```python
from build123d import *

# Parameters (mm, degrees)
F0_R      = 3.175
F1_DEPTH  = 38.1
F3_R      = 9.525
F4_DEPTH  = 3.175
F5_R      = 3.048
F6_DEPTH  = 92.0760001
F8_DEPTH  = 6.3510001273
F12_R     = 0.79375
F15_ANGLE = 180


with BuildPart() as f1:
    # F0 (on Top) → F1 (new body, symmetric)
    with BuildSketch(Plane.XY):
        Circle(F0_R)
    extrude(amount=F1_DEPTH, both=True)

    # F3 (on Right) → F4 (join, symmetric)
    with BuildSketch(Plane.YZ):
        with Locations((0, -44.45)):
            Circle(F3_R)
    extrude(amount=F4_DEPTH, both=True)

    # F5 (on face) → F6 (cut, through all)
    with BuildSketch(Plane.XY.offset(38.1)):
        Circle(F5_R)
    extrude(amount=-F6_DEPTH, mode=Mode.SUBTRACT)

    # F7 (on face) → F8 (cut, through all)
    with BuildSketch(Plane.YZ.offset(3.175)):
        with BuildLine():
            ThreePointArc((0, -35.56), (-6.2861792847, -50.7361792847), (8.89, -44.45))
            ThreePointArc((8.89, -44.45), (6.2861792847, -38.1638207153), (0, -35.56))
        make_face()
    extrude(amount=-F8_DEPTH, mode=Mode.SUBTRACT)

    # F12 (on offset) → F13 (join, up to the next surface of F1)
    with BuildSketch(Plane.XZ.offset(9.525)):
        with Locations((0, -40.48125)):
            Circle(F12_R)
        with Locations((0, -48.41875)):
            Circle(F12_R)
    extrude(until=Until.NEXT, dir=(0, 1, 0))

    # F14 (on face) → F15 (revolve)
    with BuildSketch(Plane.XZ.offset(9.525)):
        with BuildLine():
            ThreePointArc((0, -41.275), (0.5612660076, -41.0425160076), (0.79375, -40.48125))
            ThreePointArc((0.79375, -40.48125), (-0.5612660076, -39.9199839924), (0, -41.275))
        make_face()
    revolve(axis=Axis((2.719247248, -9.525, -44.45), (1, 0, 0)), revolution_arc=F15_ANGLE)


solid = f1.part
```
Here's how the part is built. I have some questions about the finished solid (model axes, mm). Round coordinates to 2 decimals unless told otherwise and drop trailing zeros. Write each loop counter-clockwise with the first axis right and the second up, starting at its lowest first coordinate (ties: lowest second). Pieces come first, ordered by that corner, then holes. Notation, with made-up numbers: M -27.5,-19.75 L -11.5,-19.75 A24 cw -11.5,-6.75 Z; hole C 14,59 d6. An arc over 180 degrees is marked long. Answer as CSV lines item,"result". Start each with the question number.
1. Thinking about a two-plate mould opening in X: for faces 1 (the cylindrical face through (-2.247, 2.06, -53.383)), 2 (the flat face through (3.175, -8, -40)), 3 (the flat face through (-3.175, -8, -40)), which applies, released by +X, released by -X, zero draft, split by the parting line, or undercut?
2. I need wall thicknesses on probe 1 along Y at (x, z) = (-1.5, -44.45) (3 decimals); probe 2 along X at (y, z) = (2.25, 19). Which ranges of each line are inside material? Lowest first, please.
3. I'm going to push flat-ended pins straight in: pin 1 Ø3 at (x, z) = (0.5, 25) entering from -Y (3 decimals); pin 2 Ø1 at (x, y) = (-2, 4) entering from -Z; pin 3 Ø1.5 at (x, y) = (-2, -4) entering from -Z. Where does each tip first touch, or does it pass through?
4. Suppose I cut it at A-A on y = -4.75. Write out the boundary of the cut face in (x, z) (3 decimals).
5. Suppose I cut it at B-B on y = 1.25. Write out the boundary of the cut face in (x, z) (3 decimals).
6. Suppose I cut it at C-C on z = 31. Write out the boundary of the cut face in (x, y) (3 decimals), then the cut area to 3 significant figures.
Check result:
1,face 1,"undercut"
1,face 2,"released by +X"
1,face 3,"released by -X"
2,probe 1,"y = -9.525 to -8.89, 8.89 to 9.525"
2,probe 2,"x = -2.24 to -2.06, 2.06 to 2.24"
3,pin 1,"stops at y = -3.175"
3,pin 2,"stops at z = -53.31"
3,pin 3,"stops at z = -53.4"
4,outline,"M -3.175,-52.706 L 3.175,-52.706 L 3.175,-51.965 L -3.175,-51.965 Z; M -3.175,-36.935 L 3.175,-36.935 L 3.175,-36.194 L -3.175,-36.194 Z"
5,outline,"M -3.175,-53.893 L -2.78,-53.893 L -2.78,-53.252 L -3.175,-53.252 Z; M -3.175,-35.648 L -2.78,-35.648 L -2.78,38.1 L -2.919,38.1 L -2.919,-35.007 L -3.175,-35.007 Z; M 2.78,-53.893 L 3.175,-53.893 L 3.175,-53.252 L 2.78,-53.252 Z; M 2.78,-35.648 L 3.175,-35.648 L 3.175,-35.007 L 2.919,-35.007 L 2.919,38.1 L 2.78,38.1 Z"
6,outline,"C 0,0 d6.35; hole C 0,0 d6.096"
6,area,"2.48 mm2"
